from build123d import *

# Parameters (mm, degrees)
F0_R          = 25.4
F0_R_2        = 12.7
F1_DEPTH      = 76.2
F3_DEPTH      = 25.401
F3_DEPTH_BACK = 25.4
F5_DEPTH      = 25.4
F5_DEPTH_BACK = 12.7
F6_W          = 25.4
F6_H          = 14.4014773719
F7_DEPTH      = 76.201
F8_DEPTH      = 76.201


with BuildPart() as f1:
    # F0 (on Right) → F1 (new body)
    with BuildSketch(Plane.YZ):
        Circle(F0_R)
        Circle(F0_R_2, mode=Mode.SUBTRACT)
    extrude(amount=F1_DEPTH)

    # F2 (on Front) → F3 (cut, two sides)
    with BuildSketch(Plane.XZ) as f3_sk:
        Polygon((76.2, 25.4), (50.8, 25.4), (50.8, -9.525), (63.5, -9.525), (63.5, 9.525), (76.2, 9.525), align=None)
    extrude(amount=-F3_DEPTH, mode=Mode.SUBTRACT)
    extrude(f3_sk.sketch, amount=F3_DEPTH_BACK, mode=Mode.SUBTRACT)

    # F4 (on Front) → F5 (join, two sides)
    with BuildSketch(Plane.XZ) as f5_sk:
        Polygon((31.75, 0), (0, 50.8), (0, 0), align=None)
    extrude(amount=-F5_DEPTH)
    extrude(f5_sk.sketch, amount=F5_DEPTH_BACK)

    # F6 (on face) → F7 (cut, through all)
    with BuildSketch(Plane(origin=(0, 0, 0), x_dir=(0, -1, 0), z_dir=(-1, 0, 0))):
        with Locations((0, 43.599261314)):
            Rectangle(F6_W, F6_H)
    extrude(amount=-F7_DEPTH, mode=Mode.SUBTRACT)

    # F0 (on Right) → F8 (cut, through all)
    with BuildSketch(Plane.YZ):
        Circle(F0_R_2)
    extrude(amount=F8_DEPTH, mode=Mode.SUBTRACT)


solid = f1.part
Input: part model. Units: mm. Frame: model coordinates. A direction names the side the tool comes from. Give positions to 0.01 mm unless a question says otherwise; leave off trailing zeros. Loops run counter-clockwise (first coordinate to the right, second up) from the corner with the lowest first, then second, coordinate; pieces in that order, holes last. Notation, with made-up numbers: (12, 43) -> (60, 43) arc R12 ccw to (60, 58) -> close; hole circle Ø5 at (87.25, 43). An arc over 180 degrees is marked (long way). Answer as a JSON object with one key per item and string values. Group by question number.
Item 1: Cut plane C-C, the plane y = 0. Return the cut outline in (x, z) (3 decimals).
Item 2: Line query: probe 1 along Z at (x, y) = (45, 0); probe 2 along X at (y, z) = (23, 7). Output: solid intervals per line, ascending.
Item 3: Pull-direction query (X, two-part tool) for faces 1 (the flat face through (70, -16, 9.525)), 2 (the flat face through (57, -16, -9.525)), 3 (the flat face through (12.57, 10.32, 30.69)), 4 (the flat face through (50.8, 5, 12)); classes: released by +X, released by -X, zero draft, split by the parting line, or undercut.
Item 4: Cut plane B-B, the plane x = 45.5. Return the cut outline in (y, z).
Item 5: Pin query (flat end, axial travel): P1, Ø2, axis at x = 38.5, y = -7, coming from the +Z side; P2, Ø11.5, axis at x = 11, z = 29.5, coming from the -Y side; P3, Ø3, axis at x = 49.5, y = -6, coming from the +Z side. Return the tip coordinate at first contact, or that it passes through.
Item 6: Reachability of faces 5 (the flat face through (3, 12.7, 42)), 6 (the flat face through (76.2, 5, -12)), 7 (the flat face through (63.5, -19, 0)), 8 (the flat face through (70, 16, 9.525)) from +Z, -Z, +X, -X, +Y, -Y: full face, straight path, thin tool, end or side. Return the list, or none.
Item 7: Cut plane D-D, the plane y = 20.5. Return the cut outline in (x, z) (3 decimals).
Item 8: Cut plane A-A, the plane z = 1.5. Return the cut outline in (x, y).
Checks:
{
 "1": {"outline": "(0, -25.4) -> (76.2, -25.4) -> (76.2, -12.7) -> (0, -12.7) -> close; (0, 12.7) -> (50.8, 12.7) -> (50.8, 25.4) -> (15.875, 25.4) -> (9.001, 36.399) -> (0, 36.399) -> close"},
 "2": {"probe 1": "z = -25.4 to -12.7, 12.7 to 25.4", "probe 2": "x = 0 to 50.8, 63.5 to 76.2"},
 "3": {"face 1": "zero draft", "face 2": "undercut", "face 3": "released by +X", "face 4": "undercut"},
 "4": {"outline": "circle Ø50.8 at (0, 0); hole circle Ø25.4 at (0, 0)"},
 "5": {"P1": "stops at z = 24.68", "P2": "stops at y = -12.7", "P3": "stops at z = 25"},
 "6": {"face 5": "+Z, +X, -X, -Y", "face 6": "+Z, -Z, +X, +Y, -Y", "face 7": "+Z, +Y, -Y", "face 8": "+Z, +X, +Y, -Y"},
 "7": {"outline": "(0, -14.997) -> (76.2, -14.997) -> (76.2, 9.525) -> (63.5, 9.525) -> (63.5, -9.525) -> (50.8, -9.525) -> (50.8, 14.997) -> (22.377, 14.997) -> (0, 50.8) -> close"},
 "8": {"outline": "(0, -25.36) -> (50.8, -25.36) -> (50.8, -12.61) -> (0, -12.61) -> close; (0, 12.61) -> (50.8, 12.61) -> (50.8, 25.36) -> (30.81, 25.36) -> (30.81, 25.4) -> (0, 25.4) -> close; (63.5, -25.36) -> (76.2, -25.36) -> (76.2, -12.61) -> (63.5, -12.61) -> close; (63.5, 12.61) -> (76.2, 12.61) -> (76.2, 25.36) -> (63.5, 25.36) -> close"}
}
